Source: three-view drawing plus pictorial views. Frame: mm from the lowest corner of the part. A direction names the side the tool comes from. Give positions to 0.01 mm unless a question says otherwise; leave off trailing zeros. Loops run counter-clockwise (first coordinate to the right, second up) from the corner with the lowest first, then second, coordinate; pieces in that order, holes last. Notation, with made-up numbers: (2.25, -13.75) - (11.25, -13.75) arc R8 cw to (11.25, -0.75) - close; hole circle Ø10 at (26.25, 65). An arc over 180 degrees is marked (long way). One line per item, written item: value.
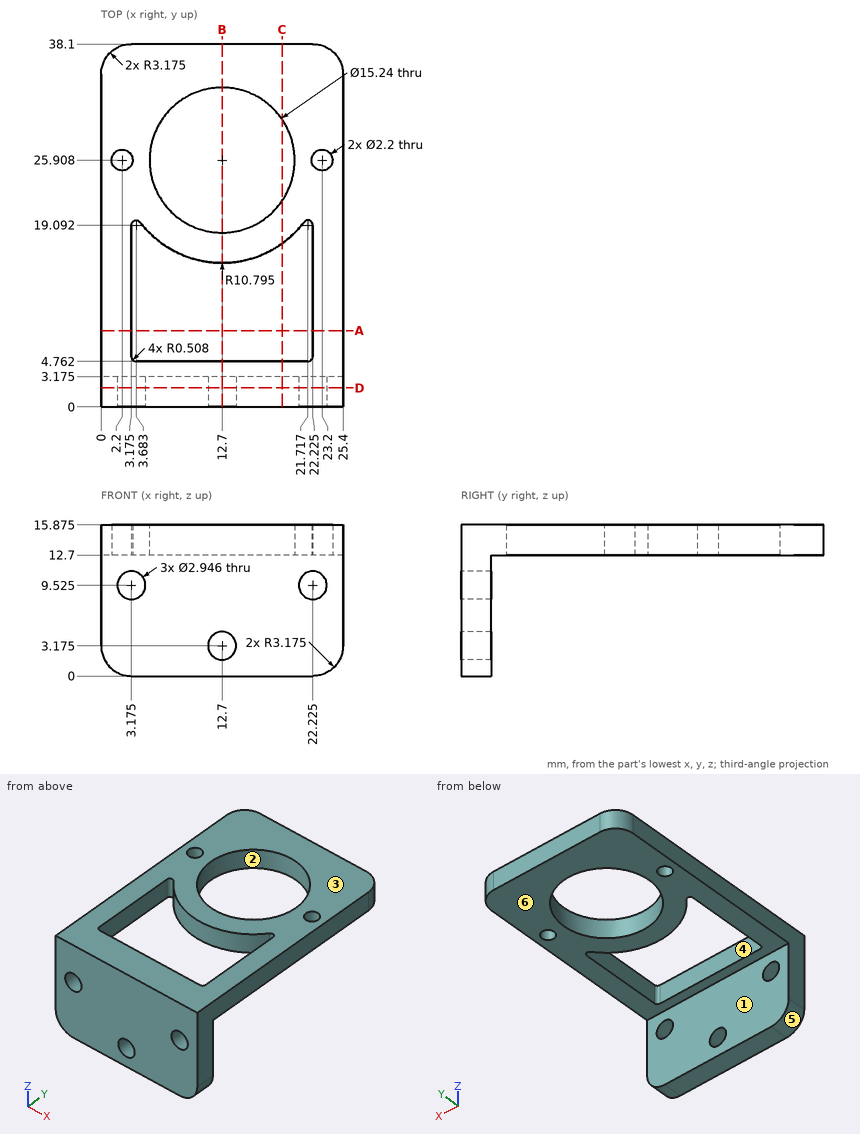
Item 1: Section A-A, the plane y = 8. Output: boundary loops of the cut face in (x, z) (1 decimal).
Verdict:
outline: (0, 12.7) - (3.2, 12.7) - (3.2, 15.9) - (0, 15.9) - close; (22.2, 12.7) - (25.4, 12.7) - (25.4, 15.9) - (22.2, 15.9) - close
Item 2: Draft query along Y for the marked faces 1, 2 and 3. Return one class per face: pulls with the +Y half, pulls with the -Y half, needs draft (parallel to the pull), parting line crosses it, or undercut.
Verdict:
face 1: pulls with the +Y half
face 2: undercut
face 3: needs draft
Item 3: Material intervals for L1, parallel to Y at x = 14.25, z = 12.75 (1 decimal); L2, parallel to X at y = 19, z = 14 (1 decimal); L3, parallel to X at y = 8.5, z = 13.75 (1 decimal), sorted ascending.
Verdict:
L1: y = 0 to 4.8, 15.2 to 18.4, 33.4 to 38.1
L2: x = 0 to 3.2, 4.4 to 9.5, 15.9 to 21, 22.2 to 25.4
L3: x = 0 to 3.2, 22.2 to 25.4
Item 4: Section C-C, the plane x = 19. Output: boundary loops of the cut face in (y, z) (1 decimal).
Verdict:
outline: (0, 0) - (3.2, 0) - (3.2, 12.7) - (4.8, 12.7) - (4.8, 15.9) - (0, 15.9) - close; (17.1, 12.7) - (21.6, 12.7) - (21.6, 15.9) - (17.1, 15.9) - close; (30.2, 12.7) - (38.1, 12.7) - (38.1, 15.9) - (30.2, 15.9) - close
Item 5: Pin query (flat end, axial travel): P1, Ø4, axis at x = 21, y = 23, coming from the -Z side; P2, Ø1.5, axis at x = 18, z = 2.5, coming from the +Y side (1 decimal). Return the tip coordinate at first contact, or that it passes through.
Verdict:
P1: stops at z = 12.7
P2: stops at y = 3.2
Item 6: Section B-B, the plane x = 12.7. Output: boundary loops of the cut face in (y, z) (1 decimal).
Verdict:
outline: (0, 0) - (3.2, 0) - (3.2, 1.7) - (0, 1.7) - close; (0, 4.6) - (3.2, 4.6) - (3.2, 12.7) - (4.8, 12.7) - (4.8, 15.9) - (0, 15.9) - close; (15.1, 12.7) - (18.3, 12.7) - (18.3, 15.9) - (15.1, 15.9) - close; (33.5, 12.7) - (38.1, 12.7) - (38.1, 15.9) - (33.5, 15.9) - close
Item 7: Section D-D, the plane y = 2. Count the separate pieces of the cut face and the enclosed holes in it.
Verdict:
separate pieces: 1
enclosed holes: 3
Item 8: Access query for the marked faces 4, 5 and 6. Directions: +Z, -Z, +X, -X, +Y, -Y. A direction counts if a zero-diameter tool reaches every point of the face in a straight line with its end or side. Return the directions, or none.
Verdict:
face 4: +Z, -Z
face 5: -Z, -X, +Y, -Y
face 6: -Z, +X, -X, +Y
